Can you work these out from the model? Positions are in its coordinate system, mm. Face numbers are marked on the shaded views. Give positions to 0.01 mm unless a question says otherwise; leave off trailing zeros. Loops run counter-clockwise (first coordinate to the right, second up) from the corner with the lowest first, then second, coordinate; pieces in that order, holes last. Notation, with made-up numbers: (-16, 43) -> (-4, 43) arc R14 cw to (-4, 69) -> close; hole circle Ø11 at (-25.5, 84.5). An arc over 180 degrees is marked (long way). Use CSV: the item, a comma, the result in double quotes.
from build123d import *

# Parameters (mm, degrees)
F0_R     = 1.651
F1_DEPTH = 5


with BuildPart() as f1:
    # F0 (on Front) → F1 (new body)
    with BuildSketch(Plane.XZ):
        with BuildLine():
            Line((0, 0), (-27.94, 0))
            Line((-27.94, 0), (-27.94, -22.86))
            ThreePointArc((-27.94, -22.86), (-26.080128, -27.350128), (-21.59, -29.21))
            Line((-21.59, -29.21), (-6.35, -29.21))
            ThreePointArc((-6.35, -29.21), (-1.859872, -27.350128), (0, -22.86))
            Line((0, -22.86), (0, 0))
        make_face()
        with Locations((-25.4, -6.35)):
            Circle(F0_R, mode=Mode.SUBTRACT)
        with Locations((-2.54, -6.35)):
            Circle(F0_R, mode=Mode.SUBTRACT)
    extrude(amount=F1_DEPTH)


solid = f1.part
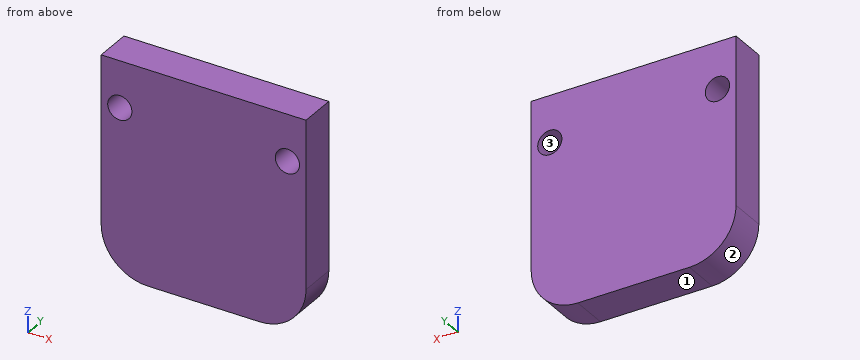
(1) Will these pins go through, and if not, where does the flat tip stop? pin 1 Ø1.5 at (x, y) = (-24, -2.5) entering from -Z; pin 2 Ø2 at (x, y) = (-19.5, -2) entering from +Z; pin 3 Ø2.5 at (x, z) = (-2.54, -6.35) entering from +Y.
Answer sheet:
pin 1,"stops at z = -28.99"
pin 2,"stops at z = 0"
pin 3,"passes through"
(2) If we section it at A-A, the plane z = -6.35: Write out the boundary of the cut face in (x, y).
Answer sheet:
outline,"(-27.94, -5) -> (-27.05, -5) -> (-27.05, 0) -> (-27.94, 0) -> close; (-23.75, -5) -> (-4.19, -5) -> (-4.19, 0) -> (-23.75, 0) -> close; (-0.89, -5) -> (0, -5) -> (0, 0) -> (-0.89, 0) -> close"
(3) If I drill on L1, parallel to Z at x = -25.4, y = -3.4; L2, parallel to Z at x = -2, y = -2.3; L3, parallel to X at y = -0.6, z = -5.25, over which ranges is the centre line in solid material (lowest first)? Write a range as from..to.
Answer sheet:
L1,"z = -27.94..-8, -4.7..0"
L2,"z = -27.49..-7.91, -4.79..0"
L3,"x = -27.94..-26.63, -24.17..-3.77, -1.31..0"
(4) If we section it at C-C, the plane x = -2.54: Write out the boundary of the cut face in (y, z).
Answer sheet:
outline,"(-5, -27.94) -> (0, -27.94) -> (0, -8) -> (-5, -8) -> close; (-5, -4.7) -> (0, -4.7) -> (0, 0) -> (-5, 0) -> close"
(5) If we section it at D-D, the plane x = -26: Write out the boundary of the cut face in (y, z).
Answer sheet:
outline,"(-5, -27.43) -> (0, -27.43) -> (0, -7.89) -> (-5, -7.89) -> close; (-5, -4.81) -> (0, -4.81) -> (0, 0) -> (-5, 0) -> close"
(6) If we section it at B-B, the plane y = -4.25: Write out the boundary of the cut face in (x, z), then the cut area to 3 significant figures.
Answer sheet:
outline,"(-27.94, -22.86) arc R6.35 ccw to (-21.59, -29.21) -> (-6.35, -29.21) arc R6.35 ccw to (0, -22.86) -> (0, 0) -> (-27.94, 0) -> close; hole circle Ø3.3 at (-25.4, -6.35); hole circle Ø3.3 at (-2.54, -6.35)"
area,"782 mm2"
(7) We'd pull the mould along X, two halves only. Please class the marked faces 1, 2 and 3: released by +X, released by -X, zero draft, split by the parting line, or undercut.
Answer sheet:
face 1,"zero draft"
face 2,"released by -X"
face 3,"undercut"
